```python
from build123d import *

# Parameters (mm, degrees)
F0_W     = 1244.6
F0_H     = 177.8
F1_DEPTH = 50.8
F2_SIZE2 = 38.1
F2_SIZE  = 38.1


with BuildPart() as f1:
    # F0 (on Top) → F1 (new body)
    with BuildSketch(Plane.XY):
        with Locations((622.3, 88.9)):
            Rectangle(F0_W, F0_H)
    extrude(amount=F1_DEPTH)

    # F2
    f2_edges = [f1.edges().sort_by_distance(p)[0] for p in [
        (622.3, 0, 50.8),
        (622.3, 177.8, 50.8),
    ]]
    chamfer(f2_edges, length=F2_SIZE, length2=F2_SIZE2)


solid = f1.part
```
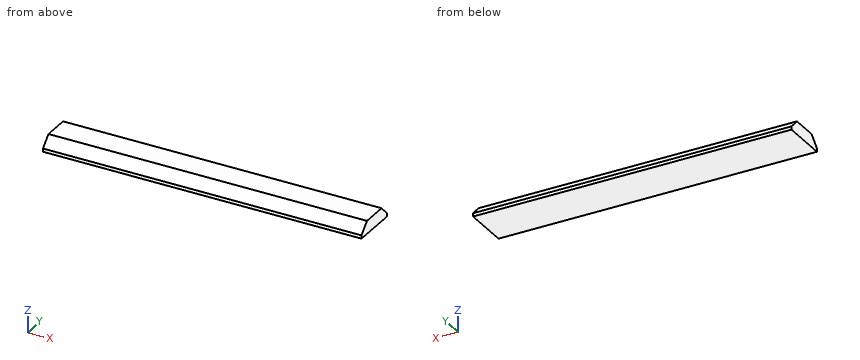
CAD build for the part. Positions are in the model's coordinates, mm. Round coordinates to 2 decimals unless told otherwise and drop trailing zeros. Order: outer loops, then holes, each group sorted by start corner. A loop starts at its lowest first (then second) coordinate and runs counter-clockwise, first axis right, second up.
Item 1: Pin check, flat tips, straight feed: pin 1 (6 mm diameter, centred on y = 74, z = 41, fed in from -X); pin 2 (12 mm diameter, centred on x = 768.5, z = 19.5, fed in from -Y). Stop position of each tip, or through.
Item 2: Saw through at B-B on z = 38.5. Write the cut outline in (x, y), then the cut area to 3 significant figures.
Item 3: Probe line 1 along Y through (x, z) = (70, 24.5); line 2 along Z through (x, y) = (315.5, 142.5); line 3 along Z through (x, y) = (265, 154). List the from-to ranges inside material, lowest first.
Item 4: Saw through at A-A on x = 787. Write the cut outline in (y, z).
Item 5: Saw through at C-C on y = 167. Write the cut outline in (x, z).
Reported:
1. pin 1: stops at x = 0
1. pin 2: stops at y = 0.8
2. outline: (0, 25.8) - (1244.6, 25.8) - (1244.6, 152) - (0, 152) - close
2. area: 157,000 mm2
3. line 1: y = 11.8 to 166
3. line 2: z = 0 to 48
3. line 3: z = 0 to 36.5
4. outline: (0, 0) - (177.8, 0) - (177.8, 12.7) - (139.7, 50.8) - (38.1, 50.8) - (0, 12.7) - close
5. outline: (0, 0) - (1244.6, 0) - (1244.6, 23.5) - (0, 23.5) - close
